```python
from build123d import *

# Parameters (mm, degrees)
F0_R     = 9.525
F1_DEPTH = 44.45
F3_DEPTH = 25.4


with BuildPart() as f1:
    # F0 (on Top) → F1 (new body)
    with BuildSketch(Plane.XY):
        with BuildLine():
            Line((88.9, 19.05), (0, 19.05))
            ThreePointArc((0, 19.05), (-13.470384, -13.470384), (19.05, 0))
            ThreePointArc((19.05, 0), (19.043512, 0.222277), (19.04481, 0.444644))
            ThreePointArc((19.04481, 0.444644), (20.313858, 4.107427), (23.475712, 6.35))
            ThreePointArc((23.475712, 6.35), (25.393079, 6.646389), (27.310446, 6.35))
            Line((27.310446, 6.35), (88.9, 6.35))
            Line((88.9, 6.35), (88.9, 19.05))
        make_face()
        Circle(F0_R, mode=Mode.SUBTRACT)
        with BuildLine():
            ThreePointArc((19.04481, 0.444644), (19.043512, 0.222277), (19.05, 0))
            ThreePointArc((19.05, 0), (19.048702, 0.222337), (19.04481, 0.444644))
        make_face()
        with BuildLine():
            ThreePointArc((27.310446, 6.35), (25.393079, 6.646389), (23.475712, 6.35))
            Line((23.475712, 6.35), (27.310446, 6.35))
        make_face()
    extrude(amount=F1_DEPTH)

    # F2 (on face) → F3 (cut)
    with BuildSketch(Plane.XZ.offset(-6.35)):
        with BuildLine():
            Line((88.9, 14.2875), (88.9, 30.1625))
            Line((88.9, 30.1625), (38.1, 30.1625))
            ThreePointArc((38.1, 30.1625), (30.1625, 22.225), (38.1, 14.2875))
            Line((38.1, 14.2875), (88.9, 14.2875))
        make_face()
        with BuildLine():
            Line((88.9, 34.925), (88.9, 44.45))
            Line((88.9, 44.45), (79.375, 44.45))
            ThreePointArc((79.375, 44.45), (86.110192, 41.660192), (88.9, 34.925))
        make_face()
        with BuildLine():
            Line((88.9, 0), (88.9, 9.525))
            ThreePointArc((88.9, 9.525), (86.110192, 2.789808), (79.375, 0))
            Line((79.375, 0), (88.9, 0))
        make_face()
    extrude(amount=-F3_DEPTH, mode=Mode.SUBTRACT)


solid = f1.part
```
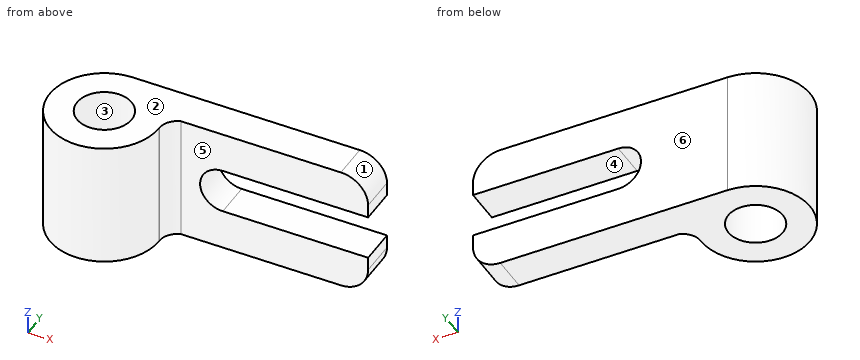
Model file for the job. Use its own axes, mm. Face numbers are marked on the shaded views. A direction names the side the tool comes from. Coordinates: 2 decimals unless noted, no trailing zeros. Write each loop counter-clockwise with the first axis right and the second up, starting at its lowest first coordinate (ties: lowest second). Pieces come first, ordered by that corner, then holes. Notation, with made-up numbers: (-35.75, -6) - (-27.75, -6) arc R38 ccw to (-27.75, 32) - close; hole circle Ø3 at (-37.5, 20). An arc over 180 degrees is marked (long way). Use a Markdown table: item, result. Add a question column.
Item 1: Drill centre lines: line 1 along Y through (x, z) = (0, 31) (3 decimals); line 2 along X through (y, z) = (-4.5, 4.5); line 3 along Y through (x, z) = (3.5, 30). Where is each one in solid material? Low to high.
Item 2: Two-plate mould, pull along X, no slides. Class the marked faces 1, 2 and 3: pulls with the +X half, pulls with the -X half, needs draft (parallel to the pull), parting line crosses it, or undercut.
Item 3: 3-axis set-ups, long thin cutter, end or side, ignore diameter. For the marked faces 4, 5 and 6: which of +Z, -Z, +X, -X, +Y, -Y reach the whole face in a straight line?
Item 4: Band-saw the part on C-C, the plane z = 38.5. Write the cut outline in (x, y) (3 decimals).
Item 5: Band-saw the part on D-D, the plane y = -14. Write the cut outline in (x, z).
Item 6: Band-saw the part on B-B, the plane y = 3.5. Write the cut outline in (x, z).
Item 7: Band-saw the part on A-A, the plane x = 56.5. Write the cut outline in (y, z), and give its area (3 significant figures).
Item 8: Drop flat-ended pins along their axis: pin 1 (1.5 mm diameter, centred on y = 10.5, z = 14, fed in from -X); pin 2 (13.5 mm diameter, centred on x = 41, z = 12, fed in from -Y); pin 3 (4 mm diameter, centred on y = -2.5, z = 37.5, fed in from +X). Give the stop position or say it passes through.
A:
| question | item | result |
|---|---|---|
| 1 | line 1 | y = -19.05 to -9.525, 9.525 to 19.05 |
| 1 | line 2 | x = -18.51 to -8.39, 8.39 to 18.51 |
| 1 | line 3 | y = -18.73 to -8.86, 8.86 to 19.05 |
| 2 | face 1 | pulls with the +X half |
| 2 | face 2 | needs draft |
| 2 | face 3 | undercut |
| 3 | face 4 | +X, +Y, -Y |
| 3 | face 5 | +Z, -Z, +X, -Y |
| 3 | face 6 | +Z, -Z, +X, -X, +Y |
| 4 | outline | (0, 19.05) arc R19.05 ccw (long way) to (19.05, 0) arc R19.056 ccw to (19.045, 0.445) arc R6.35 cw to (23.476, 6.35) - (88.204, 6.35) - (88.204, 19.05) - close; hole circle Ø19.05 at (0, 0) |
| 5 | outline | (-12.92, 0) - (12.92, 0) - (12.92, 44.45) - (-12.92, 44.45) - close |
| 6 | outline | (-18.73, 0) - (-8.86, 0) - (-8.86, 44.45) - (-18.73, 44.45) - close; (8.86, 0) - (19.91, 0) - (19.91, 44.45) - (8.86, 44.45) - close |
| 7 | outline | (6.35, 0) - (19.05, 0) - (19.05, 14.29) - (6.35, 14.29) - close; (6.35, 30.16) - (19.05, 30.16) - (19.05, 44.45) - (6.35, 44.45) - close |
| 7 | area | 363 mm² |
| 8 | pin 1 | stops at x = -16.37 |
| 8 | pin 2 | stops at y = 6.35 |
| 8 | pin 3 | stops at x = 19.04 |
